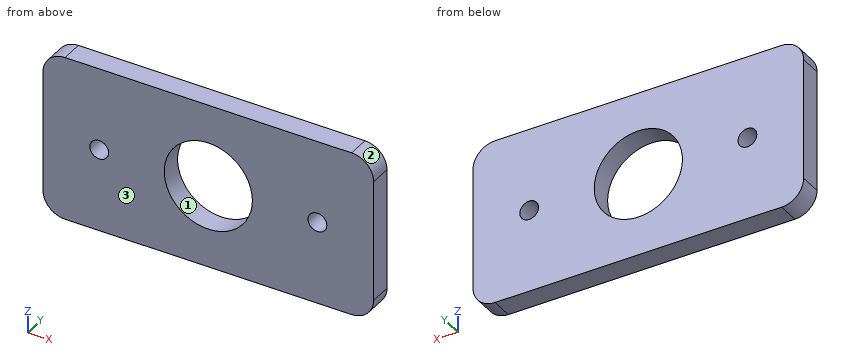
```python
from build123d import *

# Parameters (mm, degrees)
F0_W     = 150
F0_H     = 75
F0_R     = 20
F1_DEPTH = 5
F2_R     = 10
F4_D     = 8.5
F4_DEPTH = 24.5
F4_TIP   = 2.5536576309


with BuildPart() as f1:
    # F0 (on Front) → F1 (new body, symmetric)
    with BuildSketch(Plane.XZ):
        Rectangle(F0_W, F0_H)
        Circle(F0_R, mode=Mode.SUBTRACT)
    extrude(amount=F1_DEPTH, both=True)

    # F2
    f2_edges = [f1.edges().sort_by_distance(p)[0] for p in [
        (-75, 0, 37.5),
        (75, 0, 37.5),
        (75, 0, -37.5),
        (-75, 0, -37.5),
    ]]
    fillet(f2_edges, radius=F2_R)

    # F4
    with Locations(Plane.XZ.offset(5)):
        with Locations((-49.5, 0), (49.5, 0)):
            Hole(F4_D / 2, depth=F4_DEPTH)
            with Locations((0, 0, -(F4_DEPTH + F4_TIP / 2))):  # 118° drill point
                Cone(0, F4_D / 2, F4_TIP, mode=Mode.SUBTRACT)


solid = f1.part
```
CAD build for the part. Positions are in the model's coordinates, mm. Face numbers are marked on the shaded views. Coordinates: 2 decimals unless noted, no trailing zeros. Order: outer loops, then holes, each group sorted by start corner. A loop starts at its lowest first (then second) coordinate and runs counter-clockwise, first axis right, second up.
(1) Saw through at A-A, the plane x = 0. Write the cut outline in (y, z), and give its area (3 significant figures).
Solution:
outline: (-5, -37.5) - (5, -37.5) - (5, -20) - (-5, -20) - close; (-5, 20) - (5, 20) - (5, 37.5) - (-5, 37.5) - close
area: 350 mm2
(2) Saw through at B-B, the plane z = 0. Write the cut outline in (x, y), and give its area (3 significant figures).
Solution:
outline: (-75, -5) - (-53.75, -5) - (-53.75, 5) - (-75, 5) - close; (-45.25, -5) - (-20, -5) - (-20, 5) - (-45.25, 5) - close; (20, -5) - (45.25, -5) - (45.25, 5) - (20, 5) - close; (53.75, -5) - (75, -5) - (75, 5) - (53.75, 5) - close
area: 930 mm2
(3) Mould opens along X. For the marked faces 1, 2 and 3 say: released by +X, released by -X, zero draft, split by the parting line, or undercut.
Solution:
face 1: undercut
face 2: released by +X
face 3: zero draft
(4) Drill centre lines: L1, parallel to Z at x = 49.5, y = 0.75; L2, parallel to Z at x = 0, y = 1.5; L3, parallel to X at y = -3.25, z = 28. Where is each one in solid material? Low to high.
Solution:
L1: z = -37.5 to -4.25, 4.25 to 37.5
L2: z = -37.5 to -20, 20 to 37.5
L3: x = -74.99 to 74.99
(5) Saw through at C-C, the plane x = 49.5. Write the cut outline in (y, z), and give its area (3 significant figures).
Solution:
outline: (-5, -37.5) - (5, -37.5) - (5, -4.25) - (-5, -4.25) - close; (-5, 4.25) - (5, 4.25) - (5, 37.5) - (-5, 37.5) - close
area: 665 mm2
